Read the model definition and answer for the solid it produces. Units are mm, in the model's axes. Face numbers are marked on the shaded views. A direction names the side the tool comes from. Coordinates: 2 decimals unless noted, no trailing zeros. Order: outer loops, then holes, each group sorted by start corner. A loop starts at its lowest first (then second) coordinate and runs counter-clockwise, first axis right, second up. Notation, with made-up numbers: M 23,62.5 L 48,62.5 A5 ccw 48,67.5 Z; hole C 22.5,76 d8. An arc over 180 degrees is marked long. One line per question, with ' | ' between items. Start each with the question number.
1) Consider probe 1 along X at (y, z) = (16.5, 10); probe 2 along Y at (x, z) = (74.5, -27); probe 3 along X at (y, z) = (56, -81.5). Determine where each line is inside the solid, lowest interval first.
2) A tool of negligible diameter and unlimited length cuts with its end or side. For the marked faces 4 and 5, from which of +Z, -Z, +X, -X, +Y, -Y can it reach the whole face along a straight path? Write none if from no direction.
3) Find section D-D, the plane z = -46. Write down the section's boundary in (x, y), plus the area to 3 significant figures.
4) Find section B-B, the plane z = 0. Write down the section's boundary in (x, y).
5) Given P1, Ø1, axis at y = 64.5, z = -57, coming from the +X side; P2, Ø8, axis at x = -51.5, y = 87.5, coming from the +Z side; P3, Ø1.6, axis at y = 5.5, z = 93, coming from the +X side, each flat-ended and moving along its own axis, determine where each tip first touches the part or whether it passes through.
6) The mould has two halves that part along X. Classify the marked faces 1, 2 and 3: +X half, -X half, draft (parallel to the pull), parting line (faces both ways), or undercut.
7) Find section C-C, the plane y = 73. Write down the section's boundary in (x, z), plus the area to 3 significant figures.
from build123d import *

# Parameters (mm, degrees)
SKETCH1_R               = 127
BOSS_EXTRUDE1_DEPTH     = 6.35
SKETCH2_W               = 136.525
SKETCH2_H               = 187.325
SKETCH2_W_2             = 130.175
SKETCH2_H_2             = 180.975
BOSS_EXTRUDE2_DEPTH     = 180.975
CUT_EXTRUDE1_REACH      = 197.262
CUT_EXTRUDE2_REACH      = 222.663
SKETCH6_W               = 130.175
SKETCH6_H               = 180.975
CUT_EXTRUDE3_REACH      = 8.35
SKETCH7_W               = 130.175
SKETCH7_H               = 180.975
BOSS_EXTRUDE3_DEPTH     = 136.525
CUT_EXTRUDE4_DEPTH      = 136.525
SKETCH15_R              = 3.175
CUT_EXTRUDE5_DEPTH      = 6.35
CUT_EXTRUDE5_DEPTH_BACK = 142.875


with BuildPart() as part:
    # Sketch1 → Boss-Extrude1 (new body)
    with BuildSketch(Plane(origin=(0, 0, 0), x_dir=(1, 0, 0), z_dir=(0, 1, 0))):
        Circle(SKETCH1_R)
    extrude(amount=BOSS_EXTRUDE1_DEPTH)

    # Sketch2 → Boss-Extrude2 (add)
    with BuildSketch(Plane(origin=(0, 6.35, 0), x_dir=(1, 0, 0), z_dir=(0, 1, 0))):
        Rectangle(SKETCH2_W, SKETCH2_H)
        Rectangle(SKETCH2_W_2, SKETCH2_H_2, mode=Mode.SUBTRACT)
    extrude(amount=BOSS_EXTRUDE2_DEPTH)

    # Sketch3 → Cut-Extrude1 (cut, up to next)
    with BuildSketch(Plane(origin=(68.2625, 0, 0), x_dir=(0, 0, -1), z_dir=(1, 0, 0)), mode=Mode.PRIVATE) as cut_extrude1_sk1:
        with BuildLine():
            Line((-93.6625, 187.325), (93.6625, 187.325))
            Line((93.6625, 187.325), (93.6625, 6.35))
            Line((93.6625, 6.35), (87.3125, 6.35))
            ThreePointArc((87.3125, 6.35), (34.306149725, 134.318649725), (-93.6625, 187.325))
        make_face()
    cut_extrude1_tool1 = extrude(cut_extrude1_sk1.sketch, amount=-CUT_EXTRUDE1_REACH, mode=Mode.PRIVATE) & part.part
    add(cut_extrude1_tool1.solids().sort_by_distance((68.2625, 139.865797, -53.015255))[0], mode=Mode.SUBTRACT)

    # Sketch6 → Cut-Extrude2 (cut, up to next)
    with BuildSketch(Plane.XY.offset(93.6625), mode=Mode.PRIVATE) as cut_extrude2_sk1:
        with Locations((0, 96.8375)):
            Rectangle(SKETCH6_W, SKETCH6_H)
    cut_extrude2_tool1 = extrude(cut_extrude2_sk1.sketch, amount=-CUT_EXTRUDE2_REACH, mode=Mode.PRIVATE) & part.part
    add(cut_extrude2_tool1.solids().sort_by_distance((0, 96.8375, 93.6625))[0], mode=Mode.SUBTRACT)

    # Sketch7 → Cut-Extrude3 (cut, up to next)
    with BuildSketch(Plane(origin=(0, 6.35, 0), x_dir=(1, 0, 0), z_dir=(0, 1, 0)), mode=Mode.PRIVATE) as cut_extrude3_sk1:
        with Locations((0, -3.175)):
            Rectangle(SKETCH7_W, SKETCH7_H)
    cut_extrude3_tool1 = extrude(cut_extrude3_sk1.sketch, amount=-CUT_EXTRUDE3_REACH, mode=Mode.PRIVATE) & part.part
    add(cut_extrude3_tool1.solids().sort_by_distance((0, 6.35, 3.175))[0], mode=Mode.SUBTRACT)

    # Sketch10 → Boss-Extrude3 (add)
    with BuildSketch(Plane(origin=(68.2625, 0, 0), x_dir=(0, 0, -1), z_dir=(1, 0, 0))):
        with BuildLine():
            Line((-93.6625, 187.325), (-93.6625, 190.5))
            ThreePointArc((-93.6625, 190.5), (36.551213756, 136.563713756), (90.4875, 6.35))
            Line((90.4875, 6.35), (87.3125, 6.35))
            ThreePointArc((87.3125, 6.35), (34.306149725, 134.318649725), (-93.6625, 187.325))
        make_face()
    extrude(amount=-BOSS_EXTRUDE3_DEPTH)

    # Sketch12 → Cut-Extrude4 (cut)
    with BuildSketch(Plane(origin=(68.2625, 0, 0), x_dir=(0, 0, -1), z_dir=(1, 0, 0))):
        with BuildLine():
            Line((-93.6625, 6.35), (36.551213756, 136.563713756))
            ThreePointArc((36.551213756, 136.563713756), (-23.19134593, 176.482415912), (-93.6625, 190.5))
            Line((-93.6625, 190.5), (-93.6625, 6.35))
        make_face()
    extrude(amount=-CUT_EXTRUDE4_DEPTH, mode=Mode.SUBTRACT)

    # Sketch15 → Cut-Extrude5 (cut, two sides)
    with BuildSketch(Plane(origin=(68.2625, 0, 0), x_dir=(0, 0, -1), z_dir=(1, 0, 0))) as cut_extrude5_sk:
        with Locations((-93.6625, 6.35)):
            Circle(SKETCH15_R)
    extrude(amount=CUT_EXTRUDE5_DEPTH, mode=Mode.SUBTRACT)
    extrude(cut_extrude5_sk.sketch, amount=-CUT_EXTRUDE5_DEPTH_BACK, mode=Mode.SUBTRACT)


solid = part.part
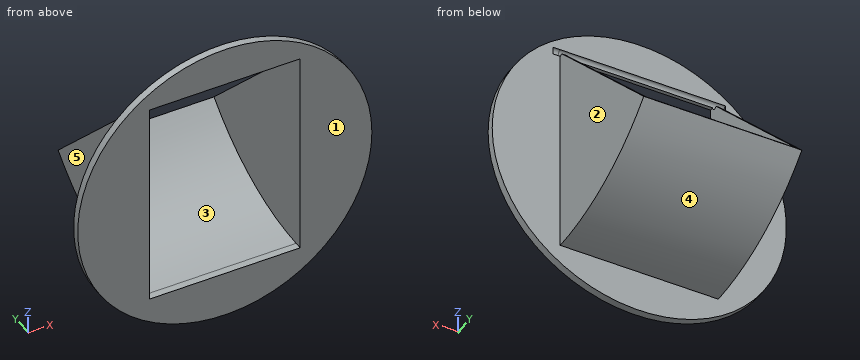
Report:
1) probe 1: x = -68.26 to -65.09, 65.09 to 68.26 | probe 2: y = 0 to 6.35 | probe 3: x = -68.26 to 68.26
2) face 4: -Z, +X, -X, +Y | face 5: +Z, -Z, -X, +Y
3) outline: M -118.38,0 L -65.09,0 L -65.09,121.44 L 65.09,121.44 L 65.09,0 L 118.38,0 L 118.38,6.35 L 68.26,6.35 L 68.26,126.37 L -68.26,126.37 L -68.26,6.35 L -118.38,6.35 Z | area: 2,080 mm^2
4) outline: M -127,0 L -65.09,0 L -65.09,100.01 L -68.26,100.01 L -68.26,6.35 L -127,6.35 Z; M 65.09,0 L 127,0 L 127,6.35 L 68.26,6.35 L 68.26,100.01 L 65.09,100.01 Z
5) P1: stops at x = 68.26 | P2: stops at z = -66.03 | P3: stops at x = 87.34
6) face 1: draft | face 2: +X half | face 3: undercut
7) outline: M -68.26,-78 L 68.26,-78 L 68.26,27.01 L 65.09,27.01 L 65.09,-74.59 L -65.09,-74.59 L -65.09,27.01 L -68.26,27.01 Z | area: 1,110 mm^2
